from build123d import *

# Parameters (mm, degrees)
SKETCH1_W           = 150
SKETCH1_H           = 225
BOSS_EXTRUDE1_DEPTH = 5
SKETCH2_R           = 1.125
CUT_EXTRUDE1_DEPTH  = 136.300591277
SKETCH3_R           = 1.275
CUT_EXTRUDE2_DEPTH  = 136.300591277
SKETCH6_W           = 20
SKETCH6_H           = 5
CUT_EXTRUDE3_DEPTH  = 136.300591277
SKETCH9_W           = 12.5
SKETCH9_H           = 65
SKETCH9_W_2         = 17.5
SKETCH9_H_2         = 12.5
CUT_EXTRUDE4_DEPTH  = 5
SKETCH10_W          = 25
SKETCH10_H          = 5
SKETCH10_W_2        = 5
SKETCH10_H_2        = 25
CUT_EXTRUDE5_DEPTH  = 5


with BuildPart() as part:
    # Sketch1 → Boss-Extrude1 (new body)
    with BuildSketch(Plane(origin=(0, 0, 0), x_dir=(1, 0, 0), z_dir=(0, 1, 0))):
        Rectangle(SKETCH1_W, SKETCH1_H)
    extrude(amount=BOSS_EXTRUDE1_DEPTH)

    # Sketch2 → Cut-Extrude1 (cut, through all)
    with BuildSketch(Plane(origin=(0, 5, 0), x_dir=(1, 0, 0), z_dir=(0, 1, 0))):
        with Locations(Location((-35.35, 82.5, 0), (0, 0, 270))):
            Circle(SKETCH2_R)
        with Locations(Location((25, 82.5, 0), (0, 0, 270))):
            Circle(SKETCH2_R)
        with Locations(Location((25, -6, 0), (0, 0, 270))):
            Circle(SKETCH2_R)
        with Locations(Location((-35.35, -6, 0), (0, 0, 270))):
            Circle(SKETCH2_R)
    extrude(amount=-CUT_EXTRUDE1_DEPTH, mode=Mode.SUBTRACT)

    # Sketch3 → Cut-Extrude2 (cut, through all)
    with BuildSketch(Plane(origin=(0, 5, 0), x_dir=(1, 0, 0), z_dir=(0, 1, 0))):
        with Locations(Location((28, -30.5, 0), (0, 0, 270))):
            Circle(SKETCH3_R)
        with Locations(Location((65, -30.5, 0), (0, 0, 270))):
            Circle(SKETCH3_R)
        with Locations(Location((65, -67.5, 0), (0, 0, 270))):
            Circle(SKETCH3_R)
        with Locations(Location((28, -67.5, 0), (0, 0, 270))):
            Circle(SKETCH3_R)
    extrude(amount=-CUT_EXTRUDE2_DEPTH, mode=Mode.SUBTRACT)

    # Sketch6 → Cut-Extrude3 (cut, through all)
    with BuildSketch(Plane(origin=(0, 5, 0), x_dir=(1, 0, 0), z_dir=(0, 1, 0))):
        with Locations((0, 103)):
            Rectangle(SKETCH6_W, SKETCH6_H)
    extrude(amount=-CUT_EXTRUDE3_DEPTH, mode=Mode.SUBTRACT)

    # Sketch9 → Cut-Extrude4 (cut)
    with BuildSketch(Plane(origin=(0, 5, 0), x_dir=(1, 0, 0), z_dir=(0, 1, 0))):
        with Locations((11.75, -57.5)):
            Rectangle(SKETCH9_W, SKETCH9_H)
        with Locations((38.75, -14.25)):
            Rectangle(SKETCH9_W_2, SKETCH9_H_2)
        with Locations((38.75, -83.75)):
            Rectangle(SKETCH9_W_2, SKETCH9_H_2)
    extrude(amount=-CUT_EXTRUDE4_DEPTH, mode=Mode.SUBTRACT)

    # Sketch10 → Cut-Extrude5 (cut)
    with BuildSketch(Plane(origin=(0, 5, 0), x_dir=(1, 0, 0), z_dir=(0, 1, 0))):
        with Locations((-55.5, -103)):
            Rectangle(SKETCH10_W, SKETCH10_H)
        with Locations((-55.5, 103)):
            Rectangle(SKETCH10_W, SKETCH10_H)
        with Locations((55.5, -103)):
            Rectangle(SKETCH10_W, SKETCH10_H)
        with Locations((55.5, 103)):
            Rectangle(SKETCH10_W, SKETCH10_H)
        with Locations((65.5, 0)):
            Rectangle(SKETCH10_W_2, SKETCH10_H_2)
        with Locations((-65.5, 0)):
            Rectangle(SKETCH10_W_2, SKETCH10_H_2)
    extrude(amount=-CUT_EXTRUDE5_DEPTH, mode=Mode.SUBTRACT)


solid = part.part
The model under review builds one solid part; all positions refer to its coordinate system, in mm. Round coordinates to 2 decimals unless told otherwise and drop trailing zeros. Loops run counter-clockwise (first coordinate to the right, second up) from the corner with the lowest first, then second, coordinate; pieces in that order, holes last. Notation, with made-up numbers: (70.5, 60) -> (88.5, 60) arc R32 cw to (88.5, 91) -> close; hole circle Ø2 at (27.25, 86.5). An arc over 180 degrees is marked (long way). Write item = value, one per line. Start each with the question number.
Item 1: Take a section at A-A on x = 14. Give the boundary of the cut face in (y, z).
Item 2: To check wall thickness, follow L1, parallel to Z at x = 7.5, y = 4.1; L2, parallel to Z at x = -61.5, y = 0.8; L3, parallel to X at y = 3.6, z = 30.5 (3 decimals). State the ranges of each line that lie inside material, in increasing order.
Item 3: Take a section at D-D on y = 2.55. Count the separate pieces of the cut face and the enclosed holes in it, plus the area to 3 significant figures.
Item 4: Insertion check: pin 1 (5 mm diameter, centred on x = -47.5, z = 80, fed in from -Y). The pin has a flat end and moves straight along its axis. Give the tip position at first contact, or say it passes through.
Item 5: Take a section at C-C on z = 1. Give the boundary of the cut face in (x, y), plus the area to 3 significant figures.
Item 6: Take a section at B-B on z = 54.5. Give the boundary of the cut face in (x, y), plus the area to 4 significant figures.
Result:
q1.outline = (0, -112.5) -> (5, -112.5) -> (5, 25) -> (0, 25) -> close; (0, 90) -> (5, 90) -> (5, 112.5) -> (0, 112.5) -> close
q2.L1 = -112.5 to -105.5, -100.5 to 25, 90 to 112.5
q2.L2 = -112.5 to -105.5, -100.5 to 100.5, 105.5 to 112.5
q2.L3 = -75 to 5.5, 18 to 26.725, 29.275 to 63.725, 66.275 to 75
q3.separate_pieces = 1
q3.enclosed_holes = 18
q3.area = 31,600 mm²
q4.pin_1 = 0
q5.outline = (-75, 0) -> (-68, 0) -> (-68, 5) -> (-75, 5) -> close; (-63, 0) -> (63, 0) -> (63, 5) -> (-63, 5) -> close; (68, 0) -> (75, 0) -> (75, 5) -> (68, 5) -> close
q5.area = 700 mm²
q6.outline = (-75, 0) -> (5.5, 0) -> (5.5, 5) -> (-75, 5) -> close; (18, 0) -> (75, 0) -> (75, 5) -> (18, 5) -> close
q6.area = 687.5 mm²
